```python
from build123d import *

# Parameters (mm, degrees)
F0_W     = 70
F0_H     = 200
F1_DEPTH = 10
F3_DEPTH = 25
F4_DEPTH = 25
F5_R     = 10
F6_R     = 10


with BuildPart() as f1:
    # F0 (on Top) → F1 (new body)
    with BuildSketch(Plane.XY):
        with Locations((13.355264, 39.517543)):
            Rectangle(F0_W, F0_H)
    extrude(amount=F1_DEPTH)

    # F2 (on face) → F3 (cut)
    with BuildSketch(Plane.XY.offset(10)):
        with BuildLine():
            ThreePointArc((13.355264, 129.517543), (7.078077, 109.517543), (13.355264, 89.517543))
            ThreePointArc((13.355264, 89.517543), (19.63245, 109.517543), (13.355264, 129.517543))
        make_face()
        with BuildLine():
            ThreePointArc((13.355264, -10.482457), (7.078077, -30.482457), (13.355264, -50.482457))
            ThreePointArc((13.355264, -50.482457), (19.63245, -30.482457), (13.355264, -10.482457))
        make_face()
        with BuildLine():
            Line((9.913476, 33.144401), (6.369316, 36.672719))
            ThreePointArc((6.369316, 36.672719), (13.355264, 19.517543), (20.341211, 36.672719))
            Line((20.341211, 36.672719), (16.797051, 33.144401))
            ThreePointArc((16.797051, 33.144401), (13.355264, 24.517543), (9.913476, 33.144401))
        make_face()
        with BuildLine():
            Line((9.913476, 53.144401), (6.369316, 56.672719))
            ThreePointArc((6.369316, 56.672719), (4.093737, 45.746055), (13.355264, 39.517543))
            ThreePointArc((13.355264, 39.517543), (23.355264, 49.517543), (13.355264, 59.517543))
            Line((13.355264, 59.517543), (13.355264, 54.517543))
            Line((13.355264, 54.517543), (13.355264, 52.517543))
            Line((13.355264, 52.517543), (15.355264, 52.517543))
            Line((15.355264, 52.517543), (15.355264, 54.100118))
            ThreePointArc((15.355264, 54.100118), (14.220155, 44.592915), (9.913476, 53.144401))
        make_face()
    extrude(amount=-F3_DEPTH, mode=Mode.SUBTRACT)

    # F2 (on face) → F4 (cut)
    with BuildSketch(Plane.XY.offset(10)):
        with BuildLine():
            ThreePointArc((13.355264, 129.517543), (7.078077, 109.517543), (13.355264, 89.517543))
            ThreePointArc((13.355264, 89.517543), (19.63245, 109.517543), (13.355264, 129.517543))
        make_face()
        with BuildLine():
            ThreePointArc((13.355264, -10.482457), (7.078077, -30.482457), (13.355264, -50.482457))
            ThreePointArc((13.355264, -50.482457), (19.63245, -30.482457), (13.355264, -10.482457))
        make_face()
        with BuildLine():
            Line((9.913476, 33.144401), (6.369316, 36.672719))
            ThreePointArc((6.369316, 36.672719), (13.355264, 19.517543), (20.341211, 36.672719))
            Line((20.341211, 36.672719), (16.797051, 33.144401))
            ThreePointArc((16.797051, 33.144401), (13.355264, 24.517543), (9.913476, 33.144401))
        make_face()
        with BuildLine():
            Line((9.913476, 53.144401), (6.369316, 56.672719))
            ThreePointArc((6.369316, 56.672719), (4.093737, 45.746055), (13.355264, 39.517543))
            ThreePointArc((13.355264, 39.517543), (23.355264, 49.517543), (13.355264, 59.517543))
            Line((13.355264, 59.517543), (13.355264, 54.517543))
            Line((13.355264, 54.517543), (13.355264, 52.517543))
            Line((13.355264, 52.517543), (15.355264, 52.517543))
            Line((15.355264, 52.517543), (15.355264, 54.100118))
            ThreePointArc((15.355264, 54.100118), (14.220155, 44.592915), (9.913476, 53.144401))
        make_face()
    extrude(amount=-F4_DEPTH, mode=Mode.SUBTRACT)

    # F5
    f5_edges = [f1.edges().sort_by_distance(p)[0] for p in [
        (48.355264, -60.482457, 5),
    ]]
    fillet(f5_edges, radius=F5_R)

    # F6
    f6_edges = [f1.edges().sort_by_distance(p)[0] for p in [
        (-21.644736, -60.482457, 5),
        (-21.644736, 139.517543, 5),
        (48.355264, 139.517543, 5),
    ]]
    fillet(f6_edges, radius=F6_R)


solid = f1.part
```
Geometry check sheet. Reference: the model listing, model coordinates, mm. A direction names the side the tool comes from. Give positions to 0.01 mm unless a question says otherwise; leave off trailing zeros. Order: outer loops, then holes, each group sorted by start corner. A loop starts at its lowest first (then second) coordinate and runs counter-clockwise, first axis right, second up. Notation, with made-up numbers: (46.25, 86) - (100.25, 86) arc R37 ccw to (100.25, 122) - close; hole circle Ø6 at (75.5, -1). An arc over 180 degrees is marked (long way). Answer in a Markdown table with one row per item. Add a question column.
Q1. Mould release check, pull along Y, two halves, no side actions. Record for faces 3 (the cylindrical face through (-18.793, 136.51, 5.07)), 4 (the flat face through (13.355, 56, 5)), 5 (the flat face through (-21.645, 38, 5)): pulls with the +Y half, pulls with the -Y half, needs draft (parallel to the pull), parting line crosses it, or undercut.
Q2. Material ranges on probe 1 along Y at (x, z) = (14.5, 3.5); probe 2 along X at (y, z) = (-31.5, 7.25); probe 3 along Y at (x, z) = (15, 8), recorded low to high. Write a range as from..to.
Q3. Cross-section at B-B, the plane y = -16.5. Enter the section's corners in (x, z), then the cut area to 3 significant figures.
Q4. Cross-section at A-A, the plane z = 3.5. Enter the section's corners in (x, y).
Q5. Tool access check on faces 1 (the flat face through (48.355, 38, 5)), 2 (the flat face through (8.17, 34.88, 5.07)). Record the directions out of +Z, -Z, +X, -X, +Y, -Y that give a thin tool (end or side, any length) a straight path to the whole face; none if there is none.
Check values:
| question | item | result |
|---|---|---|
| 1 | face 3 | pulls with the +Y half |
| 1 | face 4 | undercut |
| 1 | face 5 | needs draft |
| 2 | probe 1 | y = -60.48..-48.73, -12.24..19.58, 24.65..39.58, 44.65..52.52, 59.45..91.27, 127.76..139.52 |
| 2 | probe 2 | x = -21.64..7.09, 19.62..48.36 |
| 2 | probe 3 | y = -60.48..-47.88, -13.08..19.65, 24.8..39.65, 44.8..52.52, 59.38..92.12, 126.92..139.52 |
| 3 | outline | (-21.64, 0) - (9.99, 0) - (9.99, 10) - (-21.64, 10) - close; (16.72, 0) - (48.36, 0) - (48.36, 10) - (16.72, 10) - close |
| 3 | area | 633 mm^2 |
| 4 | outline | (-21.64, -50.48) arc R10 ccw to (-11.64, -60.48) - (38.36, -60.48) arc R10 ccw to (48.36, -50.48) - (48.36, 129.52) arc R10 ccw to (38.36, 139.52) - (-11.64, 139.52) arc R10 ccw to (-21.64, 129.52) - close; hole (6.37, 36.67) arc R10 ccw (long way) to (20.34, 36.67) - (16.8, 33.14) arc R5 cw (long way) to (9.91, 33.14) - close; hole (6.37, 56.67) arc R10 ccw (long way) to (13.36, 59.52) - (13.36, 52.52) - (15.36, 52.52) - (15.36, 54.1) arc R5 cw (long way) to (9.91, 53.14) - close; hole (13.36, -50.48) arc R35 ccw to (13.36, -10.48) arc R35 ccw to start; hole (13.36, 89.52) arc R35 ccw to (13.36, 129.52) arc R35 ccw to start |
| 5 | face 1 | +Z, -Z, +X, +Y, -Y |
| 5 | face 2 | +Z, -Z |
